Autodesk Inventor part; units mm, degrees
ref_plane "YZ Plane" through (0, 0, 0) normal (1, 0, 0) x (0, 1, 0)
ref_plane "XZ Plane" through (0, 0, 0) normal (0, 1, 0) x (-1, 0, 0)
ref_plane "XY Plane" through (0, 0, 0) normal (0, 0, 1) x (1, 0, 0)
sketch "Szkic1" plane through (0, 0, 0) normal (0, 0, 1) x (1, 0, 0)
  line L0 (0, 0.1419) -> (0, -24.3581)
  line L1 (0, -24.3581) -> (-18, -24.3581)
  line L2 (-18, -24.3581) -> (-18, -23.3581)
  line L3 (0, 0.1419) -> (-1, 0.1419)
  line L4 (-1, 0.1419) -> (-18, -23.3581)
  point P0 (0, 0)
  dimension "d0" = 24.5
  dimension "d1" = 18
  dimension "d2" = 1
  dimension "d3" = 1
extrude "Wyciągnięcie proste1" add sketch "Szkic1" along normal blind 16
sketch "Szkic2" plane through (0, -24.3581, 0) normal (1, 0, 0) x (0, 0, -1)
  line L0 (0, 24.5) -> (0, 0)
  line L1 (0, 24.5) -> (-16, 24.5)
  line L2 (-16, 0) -> (-16, 24.5)
  line L3 (0, 0) -> (-16, 0)
  point P0 (0, 24.3581)
  point P1 (-8, 11)
  dimension "d6" = 16
  dimension "d7" = 13.5
  dimension "d8" = 8
hole "Otwór1" at (0, -13.3581, 8) direction (-1, 0, 0) diameter 4 end through all
sketch "Szkic3" plane through (-18, -24.3581, 0) normal (0, -1, 0) x (1, 0, 0)
  line L0 (18, 0) -> (0, 0)
  line L1 (18, 0) -> (18, 16)
  line L2 (0, 16) -> (18, 16)
  line L3 (0, 0) -> (0, 16)
  circle A0 centre (8, 8) radius 5.05
  dimension "d16" = 10.1
  dimension "d17" = 10
  dimension "d18" = 16
  dimension "d19" = 8
extrude "Wyciągnięcie proste2" cut sketch "Szkic3" against normal blind 4.15 contours A0
sketch "Szkic4" plane through (-18, -24.3581, 0) normal (-1, 0, 0) x (0, 0, 1)
  circle A0 centre (8, 11) radius 2
  circle A1 centre (8, 11) radius 4.5
  point P0 (0, 24.3581)
  dimension "d22" = 9
extrude "Wyciągnięcie proste3" cut sketch "Szkic4" against normal blind 15
fillet "Zaokrąglenie1" radius 6 2 edges at (-18, -23.8581, 16) (-18, -23.8581, 0)
chamfer "Faza1" distance 3 angle 45 2 edges at (-0.5, 0.1419, 16) (-0.5, 0.1419, 0)
equation "\"d19\" = 0.5 * d18"
properties part number "3DP_ABS_Front_Door_Frame_Magnet_Mount"
Verification items for the finished model (mm, model axes). A direction names the side the tool comes from. Coordinates: 2 decimals unless noted, no trailing zeros. Write each loop counter-clockwise with the first axis right and the second up, starting at its lowest first coordinate (ties: lowest second). Pieces come first, ordered by that corner, then holes. Notation, with made-up numbers: M 74.5,4.5 L 132.5,4.5 A37 ccw 132.5,42.5 Z; hole C 37,19.25 d4. An arc over 180 degrees is marked long. Answer as a JSON object with one key per item and string values. Group by question number.
(1) Cross-section at A-A, the plane z = 8. Record the cut outline in (x, y).
(2) Gauge pin test, flat ends, axial feed: pin 1 (1.5 mm diameter, centred on x = -13, z = 8, fed in from +Y); pin 2 (2.5 mm diameter, centred on y = -13.36, z = 8, fed in from -X); pin 3 (6 mm diameter, centred on x = -7, z = 4.5, fed in from +Y); pin 4 (8 mm diameter, centred on y = -2.5, z = 6, fed in from -X). Record the tip position at first contact, or that the pin passes through.
(3) Cross-section at B-B, the plane y = -14.5. Record the cut outline in (x, z), and give its area (3 significant figures).
(4) Cross-section at D-D, the plane y = -21.5. Record the cut outline in (x, z).
(5) Release check for a two-part mould opening along X. For faces 1 (the face through (-7.49, -8.83, 9.67)), 2 (the face through (-1.21, -1.67, 1.19)), 3 (the face through (-5.183, -22.312, 9.517)) record: +X half, -X half, draft (parallel to the pull), parting line (faces both ways), or undercut.
(6) Material ranges on line 1 (Y direction, x = -0.55, z = 8); line 2 (Y direction, x = -6.75, z = 12); line 3 (X direction, y = -16.25, z = 4.75), recorded low to high.
(7) Cross-section at C-C, the plane x = -6. Record the cut outline in (y, z), and give its area (3 significant figures).
(8) Tool access check on faces 4 (the face through (-3, -15.3, 8.94)), 5 (the face through (0, -12, 10)), 6 (the face through (-10, -20.208, 8)). Record the directions out of +Z, -Z, +X, -X, +Y, -Y that give a thin tool (end or side, any length) a straight path to the whole face; none if there is none.
Reply:
{
 "1": {"outline": "M -18,-24.36 L -15.05,-24.36 L -15.05,-20.21 L -4.95,-20.21 L -4.95,-24.36 L 0,-24.36 L 0,-15.36 L -3,-15.36 L -3,-17.86 L -14.02,-17.86 L -18,-23.36 Z; M -7.51,-8.86 L -3,-8.86 L -3,-11.36 L 0,-11.36 L 0,0.14 L -1,0.14 Z"},
 "2": {"pin 1": "y = -17.8", "pin 2": "through", "pin 3": "y = -4.01", "pin 4": "x = -5.8"},
 "3": {"outline": "M -11.59,0 L 0,0 L 0,6.36 L -3,6.36 L -3,3.65 L -11.59,3.65 Z; M -11.59,12.35 L -3,12.35 L -3,9.64 L 0,9.64 L 0,16 L -11.59,16 Z", "area": "101 mm²"},
 "4": {"outline": "M -16.66,2.22 A6 ccw -12,0 L 0,0 L 0,16 L -12,16 A6 ccw -16.66,13.78 Z; hole C -10,8 d10.1"},
 "5": {"face 1": "-X half", "face 2": "draft", "face 3": "undercut"},
 "6": {"line 1": "-24.36 to -15.36, -11.36 to 0.14", "line 2": "-24.36 to -15.42, -11.3 to -7.81", "line 3": "-3 to 0"},
 "7": {"outline": "M -24.36,0 L -6.77,0 L -6.77,16 L -24.36,16 L -24.36,11.08 L -20.21,11.08 L -20.21,4.92 L -24.36,4.92 Z; hole C -13.36,8 d9", "area": "192 mm²"},
 "8": {"face 4": "-X", "face 5": "+Z, -Z, +X, +Y, -Y", "face 6": "-Y"}
}
